The drawing under review shows one solid part. Ordinate dimensions are in mm from its lowest x, y, z. A direction names the side the tool comes from. Coordinates: 2 decimals unless noted, no trailing zeros. Write each loop counter-clockwise with the first axis right and the second up, starting at its lowest first coordinate (ties: lowest second). Pieces come first, ordered by that corner, then holes. Notation, with made-up numbers: (-14, 10) - (43, 10) arc R28 ccw to (43, 35) - close; hole circle Ø8 at (-19, 20.25). An arc over 180 degrees is marked (long way). Put each result on its own line as item: value. Start each with the question number.
Item 1: Consider section C-C on x = 11. Give the boundary of the cut face in (y, z) (1 decimal).
Item 2: For pin 1 (1.5 mm diameter, centred on x = 13.5, y = 2, fed in from -Z) (1 decimal); pin 2 (2 mm diameter, centred on x = 7, y = 14, fed in from -Z), all flat-tipped, find the tip position at first contact; note any pin that passes through.
Item 3: To check wall thickness, follow L1, parallel to Y at x = 7, z = 5.5 (1 decimal); L2, parallel to X at y = 17.5, z = 3.25; L3, parallel to Z at x = 19, y = 15.5. State the ranges of each line that lie inside material, in increasing order. Write a range as [from, to].
Item 4: Consider section D-D on y = 16.5. Give the boundary of the cut face in (x, z).
Item 5: Machinability: for the marked faces 1 and 2, which of the approach directions +Z, -Z, +X, -X, +Y, -Y give a long, thin tool a straight path to every point of the face, cutting with its end or side? Answer none if there is none.
Item 6: Consider section A-A on z = 9.25. Give the boundary of the cut face in (x, y) (1 decimal).
Item 7: Mouldability with a two-part tool opening along Y and no side actions: class the marked faces 3, 4 and 5 as pulls with the +Y half, pulls with the -Y half, needs draft (parallel to the pull), parting line crosses it, or undercut.
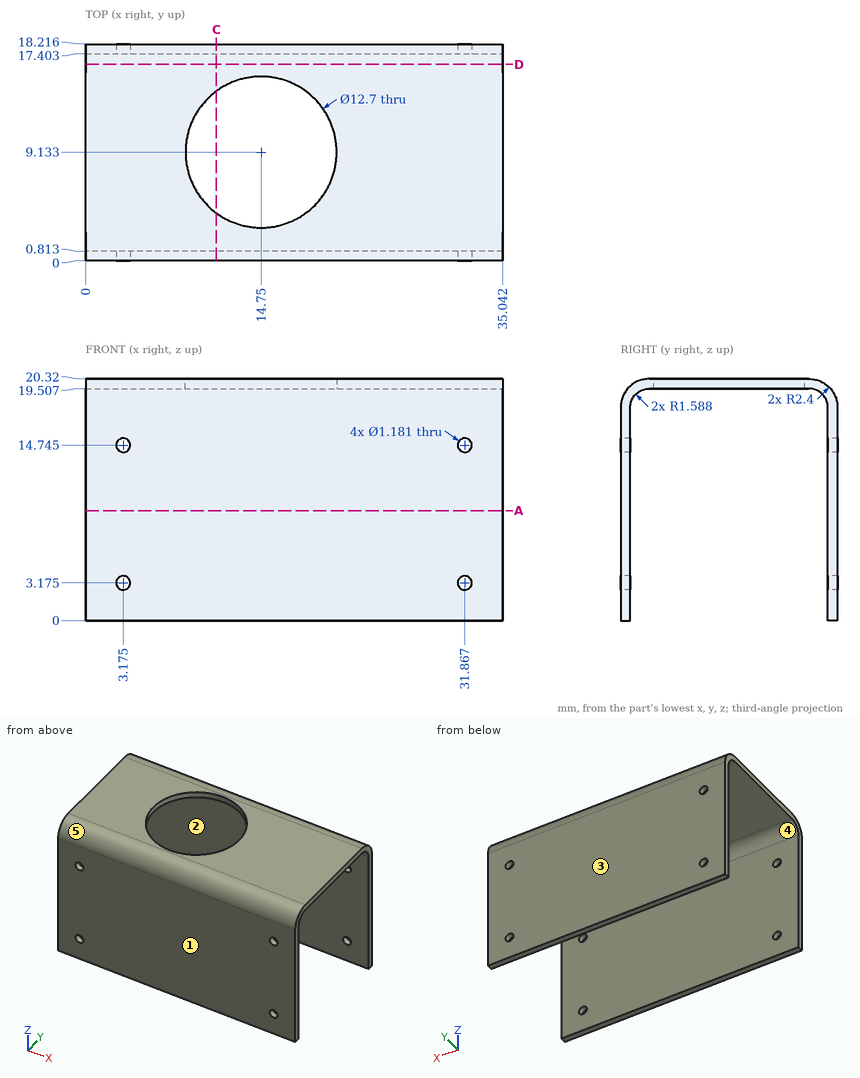
Report:
1. outline: (0, 0) - (0.8, 0) - (0.8, 17.9) arc R1.6 cw to (2.4, 19.5) - (4, 19.5) - (4, 20.3) - (2.4, 20.3) arc R2.4 ccw to (0, 17.9) - close; (14.3, 19.5) - (15.8, 19.5) arc R1.6 cw to (17.4, 17.9) - (17.4, 0) - (18.2, 0) - (18.2, 17.9) arc R2.4 ccw to (15.8, 20.3) - (14.3, 20.3) - close
2. pin 1: z = 19
2. pin 2: z = 19.51
3. L1: [0, 0.8], [17.4, 18.2]
3. L2: [0, 2.59], [3.76, 31.28], [32.45, 35.04]
3. L3: [19.51, 20.32]
4. outline: (0, 19.35) - (35.04, 19.35) - (35.04, 20.22) - (0, 20.22) - close
5. face 1: +Z, -Z, +X, -X, -Y
5. face 2: -Z, +X, -X
6. outline: (0, 0) - (35, 0) - (35, 0.8) - (0, 0.8) - close; (0, 17.4) - (35, 17.4) - (35, 18.2) - (0, 18.2) - close
7. face 3: pulls with the +Y half
7. face 4: undercut
7. face 5: pulls with the -Y half
